Build history of the part. All positions in model axes, mm. Round coordinates to 2 decimals unless told otherwise and drop trailing zeros. Order: outer loops, then holes, each group sorted by start corner. A loop starts at its lowest first (then second) coordinate and runs counter-clockwise, first axis right, second up. Notation, with made-up numbers: (82.5, -31.75) -> (103.5, -31.75) arc R5 ccw to (103.5, -27.75) -> close; hole circle Ø11 at (26.25, -14.75). An arc over 180 degrees is marked (long way). Answer as a JSON object with one key per item and string values.
from build123d import *

# Parameters (mm, degrees)
SKETCH_1_W                = 280
SKETCH_1_H                = 165
EXTRUDE_1_DEPTH           = 15
CHAMFER_1_SIZE            = 10
HOLE_WIZARD_1_D           = 13.5
HOLE_WIZARD_1_DEPTH       = 20
HOLE_WIZARD_1_CSINK_D     = 27
HOLE_WIZARD_1_CSINK_ANGLE = 92
HOLE_WIZARD_1_TIP         = 4.055809178


with BuildPart() as part:
    # 草图1 → 凸台-拉伸1 (new body)
    with BuildSketch(Plane.XY):
        Rectangle(SKETCH_1_W, SKETCH_1_H)
    extrude(amount=EXTRUDE_1_DEPTH)

    # 倒角1
    chamfer_1_edges = [part.edges().sort_by_distance(p)[0] for p in [
        (-140, 0, 15),
        (0, -82.5, 15),
        (140, 0, 15),
        (0, 82.5, 15),
    ]]
    chamfer(chamfer_1_edges, length=CHAMFER_1_SIZE)

    # 打孔尺寸(%根据)内六角花形沉头螺钉的类型1
    with Locations(Plane.XY.offset(15)):
        with Locations((-110, 50), (110, 50), (110, -50), (-110, -50)):
            CounterSinkHole(HOLE_WIZARD_1_D / 2, HOLE_WIZARD_1_CSINK_D / 2, depth=HOLE_WIZARD_1_DEPTH, counter_sink_angle=HOLE_WIZARD_1_CSINK_ANGLE)
            with Locations((0, 0, -(HOLE_WIZARD_1_DEPTH + HOLE_WIZARD_1_TIP / 2))):  # 118° drill point
                Cone(0, HOLE_WIZARD_1_D / 2, HOLE_WIZARD_1_TIP, mode=Mode.SUBTRACT)


solid = part.part
1) Flat gauge pins, fed straight in: pin 1 Ø8 at (y, z) = (36, 11) entering from +X; pin 2 Ø21.5 at (x, y) = (-110, 50) entering from +Z; pin 3 Ø2 at (x, z) = (-26, 9) entering from -Y. Where does each tip first touch, or does it go through?
Checked values:
{"pin 1": "stops at x = 138", "pin 2": "stops at z = 12.34", "pin 3": "stops at y = -79.5"}
2) Cut at D-D, the plane y = -6.5. Give the cut face in (x, z).
Checked values:
{"outline": "(-140, 0) -> (140, 0) -> (140, 5) -> (130, 15) -> (-130, 15) -> (-140, 5) -> close"}
3) Pull direction X, two halves, no side cores. Call faces 1 (the face through (103.765, -52.585, 4.181)), 2 (the face through (135, -1, 10)), 3 (the face through (-2, 82.5, 2)): pulls with the +X half, pulls with the -X half, needs draft (parallel to the pull), parting line crosses it, or undercut.
Checked values:
{"face 1": "undercut", "face 2": "pulls with the +X half", "face 3": "needs draft"}
4) Probe L1, parallel to X at y = -50, z = 2.75; L2, parallel to Y at x = 110, z = 3.25; L3, parallel to Y at x = -110, z = 6. List the from-to ranges inside material, lowest first. Write a range as from..to.
Checked values:
{"L1": "x = -140..-116.75, -103.25..103.25, 116.75..140", "L2": "y = -82.5..-56.75, -43.25..43.25, 56.75..82.5", "L3": "y = -81.5..-56.75, -43.25..43.25, 56.75..81.5"}
5) Cut at A-A, the plane y = -50. Give the cut face in (x, z).
Checked values:
{"outline": "(-140, 0) -> (-116.75, 0) -> (-116.75, 8.48) -> (-123.5, 15) -> (-130, 15) -> (-140, 5) -> close; (-103.25, 0) -> (103.25, 0) -> (103.25, 8.48) -> (96.5, 15) -> (-96.5, 15) -> (-103.25, 8.48) -> close; (116.75, 0) -> (140, 0) -> (140, 5) -> (130, 15) -> (123.5, 15) -> (116.75, 8.48) -> close"}
6) Cut at C-C, the plane z = 10.75. Give the cut face in (x, y), plus the area to 3 significant figures.
Checked values:
{"outline": "(-134.25, -76.75) -> (134.25, -76.75) -> (134.25, 76.75) -> (-134.25, 76.75) -> close; hole circle Ø18.2 at (-110, -50); hole circle Ø18.2 at (-110, 50); hole circle Ø18.2 at (110, -50); hole circle Ø18.2 at (110, 50)", "area": "40,200 mm²"}
7) Cut at B-B, the plane x = -110. Give the cut face in (y, z), plus the area to 3 significant figures.
Checked values:
{"outline": "(-82.5, 0) -> (-56.75, 0) -> (-56.75, 8.48) -> (-63.5, 15) -> (-72.5, 15) -> (-82.5, 5) -> close; (-43.25, 0) -> (43.25, 0) -> (43.25, 8.48) -> (36.5, 15) -> (-36.5, 15) -> (-43.25, 8.48) -> close; (56.75, 0) -> (82.5, 0) -> (82.5, 5) -> (72.5, 15) -> (63.5, 15) -> (56.75, 8.48) -> close", "area": "1,880 mm²"}
